from build123d import *

# Parameters (mm, degrees)
F1_DEPTH = 4


with BuildPart() as f1:
    # F0 (on Top) → F1 (new body)
    with BuildSketch(Plane.XY):
        with BuildLine():
            Line((22.830044, -28.262451), (22.830044, 46.737549))
            Line((22.830044, 46.737549), (3.330044, 46.737549))
            ThreePointArc((3.330044, 46.737549), (-2.169956, 41.237549), (-7.669956, 46.737549))
            Line((-7.669956, 46.737549), (-27.169956, 46.737549))
            Line((-27.169956, 46.737549), (-27.169956, -28.262451))
            Line((-27.169956, -28.262451), (22.830044, -28.262451))
        make_face()
        with BuildLine():
            Line((3.330044, 46.737549), (22.830044, 46.737549))
            ThreePointArc((22.830044, 46.737549), (-2.169956, 71.737549), (-27.169956, 46.737549))
            Line((-27.169956, 46.737549), (-7.669956, 46.737549))
            ThreePointArc((-7.669956, 46.737549), (-2.169956, 52.237549), (3.330044, 46.737549))
        make_face()
    extrude(amount=F1_DEPTH)


solid = f1.part
Design review of the part built by this model. Coordinates are the model's own, in mm. Round coordinates to 2 decimals unless told otherwise and drop trailing zeros. Write each loop counter-clockwise with the first axis right and the second up, starting at its lowest first coordinate (ties: lowest second). Pieces come first, ordered by that corner, then holes. Notation, with made-up numbers: M 74,-19.5 L 115,-19.5 A24 cw 115,1.5 Z; hole C -9,-37 d3. An arc over 180 degrees is marked long. One line per item, written item: value. Start each with the question number.
1. Take a section at B-B on x = -6. State the section outline as (y, z) points.
2. Take a section at D-D on x = -20. State the section outline as (y, z) points.
3. Clearance check with flat-ended pins moving along their axes: P1, Ø1, axis at y = 50, z = 0.5, coming from the -X side; P2, Ø2, axis at x = 0, z = 2, coming from the +Y side. State where each tip first meets the part, or that it passes through.
4. Take a section at A-A on z = 0.7. State the section outline as (x, y) points.
5. Draft analysis for pull direction X (two halves, no side actions). For faces 1 (the face through (22.83, 9, 2)), 2 (the face through (-1.45, 52.19, 1.97)), 3 (the face through (-3, 22, 0)), state which applies: pulls with the +X half, pulls with the -X half, needs draft (parallel to the pull), parting line crosses it, or undercut.
6. Take a section at C-C on x = 1.5. State the section outline as (y, z) points.
7. To check wall thickness, follow probe 1 along Y at (x, z) = (-2, 1.25); probe 2 along Y at (x, z) = (-4.5, 3.35); probe 3 along X at (y, z) = (48.5, 1.25). State the ranges of each line that lie inside material, in increasing order. Write a range as from..to.
Computed:
1. outline: M -28.26,0 L 42.79,0 L 42.79,4 L -28.26,4 Z; M 50.68,0 L 71.44,0 L 71.44,4 L 50.68,4 Z
2. outline: M -28.26,0 L 64.26,0 L 64.26,4 L -28.26,4 Z
3. P1: stops at x = -27.02
3. P2: stops at y = 71.71
4. outline: M -27.17,-28.26 L 22.83,-28.26 L 22.83,46.74 A25 ccw -27.17,46.74 Z; hole C -2.17,46.74 d11
5. face 1: pulls with the +X half
5. face 2: undercut
5. face 3: needs draft
6. outline: M -28.26,0 L 42.64,0 L 42.64,4 L -28.26,4 Z; M 50.83,0 L 71.47,0 L 71.47,4 L 50.83,4 Z
7. probe 1: y = -28.26..41.24, 52.23..71.74
7. probe 2: y = -28.26..41.76, 51.72..71.63
7. probe 3: x = -27.11..-7.38, 3.04..22.77
